Model file for the job. Use its own axes, mm. A direction names the side the tool comes from. Round coordinates to 2 decimals unless told otherwise and drop trailing zeros. Loops run counter-clockwise (first coordinate to the right, second up) from the corner with the lowest first, then second, coordinate; pieces in that order, holes last. Notation, with made-up numbers: M 44,72 L 59,72 A14 ccw 59,85 Z; hole C -25,51 d7. An arc over 180 degrees is marked long. Use a Markdown table: item, result. Add a question column.
Q1. Cut at A-A (x = 0). Give the cut face in (y, z), plus the area to 3 significant figures.
Q2. Tool access for faces 4 (the face through (-35, -43, 25)), 5 (the face through (52.556, 16.551, 13.922)): list every direction of +Z, -Z, +X, -X, +Y, -Y with a clear straight run to the whole face (end or side of a thin tool).
Q3. Mould opens along X. For faces 1 (the face through (-1, 1, 3.15)), 2 (the face through (-46.23, -35.44, 13.34)), 3 (the face through (-1, 1, 0)) say: +X half, -X half, draft (parallel to the pull), parting line (faces both ways), or undercut.
Q4. Pin check, flat tips, straight feed: pin 1 (3 mm diameter, centred on x = -10.5, z = 3, fed in from -Y); pin 2 (1 mm diameter, centred on y = 21, z = 15.5, fed in from +X); pin 3 (12 mm diameter, centred on x = -42.5, z = 9.5, fed in from -Y). Stop position of each tip, or through.
Q5. Probe line 1 (X direction, y = -0.5, z = 11.5); line 2 (Z direction, x = -13, y = -26). List the from-to ranges inside material, lowest first. Write a range as from..to.
Q6. Cut at C-C (z = 12). Give the cut face in (x, y).
from build123d import *

# Parameters (mm, degrees)
F0_R     = 58.25
F1_DEPTH = 25
F2_T     = -3.15
F3_R     = 2


with BuildPart() as f1:
    # F0 (on Top) → F1 (new body)
    with BuildSketch(Plane.XY):
        Circle(F0_R)
    extrude(amount=F1_DEPTH)

    # F2
    f2_openings = [f1.faces().sort_by_distance(p)[0] for p in [
        (0, 0, 25),
    ]]
    offset(amount=F2_T, openings=f2_openings)

    # F3
    f3_edges = [f1.edges().sort_by_distance(p)[0] for p in [
        (-58.25, 0, 0),
    ]]
    fillet(f3_edges, radius=F3_R)


solid = f1.part
Checked values:
| question | item | result |
|---|---|---|
| 1 | outline | M -58.25,2 A2 ccw -56.25,0 L 56.25,0 A2 ccw 58.25,2 L 58.25,25 L 55.1,25 L 55.1,3.15 L -55.1,3.15 L -55.1,25 L -58.25,25 Z |
| 1 | area | 503 mm^2 |
| 2 | face 4 | +Z, +X, -X, +Y, -Y |
| 2 | face 5 | +Z |
| 3 | face 1 | undercut |
| 3 | face 2 | parting line |
| 3 | face 3 | draft |
| 4 | pin 1 | stops at y = -57.55 |
| 4 | pin 2 | stops at x = 54.52 |
| 4 | pin 3 | stops at y = -45.4 |
| 5 | line 1 | x = -58.25..-55.1, 55.1..58.25 |
| 5 | line 2 | z = 0..3.15 |
| 6 | outline | C 0,0 d116.5; hole C 0,0 d110.2 |
